Read the model definition and answer for the solid it produces. Units are mm, in the model's axes. A direction names the side the tool comes from. Give positions to 0.01 mm unless a question says otherwise; leave off trailing zeros. Loops run counter-clockwise (first coordinate to the right, second up) from the corner with the lowest first, then second, coordinate; pieces in that order, holes last.
(1) Which of the six approach directions +Z, -Z, +X, -X, +Y, -Y give full straight-line access (tool end or side, diameter ignored) to faces 1 (the face through (-149.924, 203.805, 3.131)), 2 (the face through (-151.98, -205.86, 3.13)), 3 (the face through (88.54, 96.11, 3.22)), 4 (the face through (205.86, -151.98, 3.13))?
(2) Find section C-C, the plane y = 170. Write down the section's boundary in (x, z).
(3) Find section A-A, the plane x = 182. Write down the section's boundary in (y, z), then the cut area to 3 significant figures.
(4) Straight lines are drawn through the part: probe 1 along Y at (x, z) = (-133.35, 4.5); probe 2 along X at (y, z) = (-4.5, 1.25); probe 3 along Y at (x, z) = (-1.5, 3.5). For each, find the intervals that lie inside material, in ascending order.
(5) Find section B-B, the plane z = 3.5. State how many separate pieces and enclosed holes the cut face has, then the cut area to 3 significant figures.
(6) Each of these flat-tipped pins is pushed along its axis until it touches: P1, Ø11, axis at x = 94.29, y = 94.29, coming from the +Z side; P2, Ø3, axis at x = 44.5, z = 1, coming from the -Y side; P3, Ø1.5, axis at x = -106, z = 3, coming from the +Y side; P4, Ø3, axis at y = -180, z = 2, coming from the -X side. Where does it stop, or does it pass through?
(7) Determine the mould class of faces 5 (the face through (-251.824, -251.07, 3.131)), 6 (the face through (149.924, -203.805, 3.131)), 7 (the face through (251.824, 251.07, 3.131)) for opening direction X: pulls with the +X half, pulls with the -X half, needs draft (parallel to the pull), parting line crosses it, or undercut.
```python
from build123d import *

# Parameters (mm, degrees)
F1_DEPTH        = 6.35
F2_R            = 6.0325
F3_DEPTH        = 25.4
F3_COPIES_COUNT = 8


# Not quite as in the source:
# - a pattern or mirror of a feature is missing from the dataset's text; its kind, count and spacing are read off the source's solid


with BuildPart() as f1:
    # F0 (on Top) → F1 (new body)
    with BuildSketch(Plane.XY):
        with BuildLine():
            Line((-278.3879397531, 224.5064030267), (-131.2819155679, 77.4003788415))
            ThreePointArc((-131.2819155679, 77.4003788415), (-152.4, 0), (-131.2819155679, -77.4003788415))
            Line((-131.2819155679, -77.4003788415), (-278.3879397531, -224.5064030267))
            Line((-278.3879397531, -224.5064030267), (-224.5064030267, -278.3879397531))
            Line((-224.5064030267, -278.3879397531), (-77.4003788415, -131.2819155679))
            ThreePointArc((-77.4003788415, -131.2819155679), (0, -152.4), (77.4003788415, -131.2819155679))
            Line((77.4003788415, -131.2819155679), (224.5064030267, -278.3879397531))
            Line((224.5064030267, -278.3879397531), (278.3879397531, -224.5064030267))
            Line((278.3879397531, -224.5064030267), (131.2819155679, -77.4003788415))
            ThreePointArc((131.2819155679, -77.4003788415), (152.4, 0), (131.2819155679, 77.4003788415))
            Line((131.2819155679, 77.4003788415), (278.3879397531, 224.5064030267))
            Line((278.3879397531, 224.5064030267), (224.5064030267, 278.3879397531))
            Line((224.5064030267, 278.3879397531), (77.4003788415, 131.2819155679))
            ThreePointArc((77.4003788415, 131.2819155679), (0, 152.4), (-77.4003788415, 131.2819155679))
            Line((-77.4003788415, 131.2819155679), (-224.5064030267, 278.3879397531))
            Line((-224.5064030267, 278.3879397531), (-278.3879397531, 224.5064030267))
        make_face()
        with BuildLine():
            ThreePointArc((100.7552507667, -46.8737140403), (-108.5015964547, 24.0035245698), (111.125, 0))
            ThreePointArc((111.125, 0), (108.5015964547, -24.0035245698), (100.7552507667, -46.8737140403))
        make_face(mode=Mode.SUBTRACT)
    extrude(amount=F1_DEPTH)

    # F2 (on face) → F3 (cut)
    with BuildSketch(Plane.XY.offset(6.35)):
        with Locations((-133.35, 0)):
            Circle(F2_R)
    f3 = extrude(amount=-F3_DEPTH, mode=Mode.SUBTRACT)

    # F3_copies: F3 ×8 about axis
    f3_copies_axis = Axis((0, 0, 0), (0, 0, 1))
    for i in range(1, F3_COPIES_COUNT):
        add(f3.rotate(f3_copies_axis, i * 360 / F3_COPIES_COUNT), mode=Mode.SUBTRACT)


solid = f1.part
```
Entries:
1. face 1: +Z, -Z, +Y
1. face 2: +Z, -Z, -Y
1. face 3: +Z, -Z
1. face 4: +Z, -Z, +X
2. outline: (-223.88, 0) - (-116.12, 0) - (-116.12, 6.35) - (-223.88, 6.35) - close; (116.12, 0) - (223.88, 0) - (223.88, 6.35) - (116.12, 6.35) - close
3. outline: (-235.88, 0) - (-128.12, 0) - (-128.12, 6.35) - (-235.88, 6.35) - close; (128.12, 0) - (235.88, 0) - (235.88, 6.35) - (128.12, 6.35) - close
3. area: 1,370 mm2
4. probe 1: y = -187.23 to -79.47, -73.78 to -6.03, 6.03 to 73.78, 79.47 to 187.23
4. probe 2: x = -152.33 to -137.37, -129.33 to -111.03, 111.03 to 129.33, 137.37 to 152.33
4. probe 3: y = -152.39 to -139.19, -127.51 to -111.11, 111.11 to 127.51, 139.19 to 152.39
5. separate pieces: 1
5. enclosed holes: 9
5. area: 95,700 mm2
6. P1: passes through
6. P2: stops at y = -146.21
6. P3: stops at y = 160.63
6. P4: stops at x = -235.38
7. face 5: pulls with the -X half
7. face 6: undercut
7. face 7: pulls with the +X half
